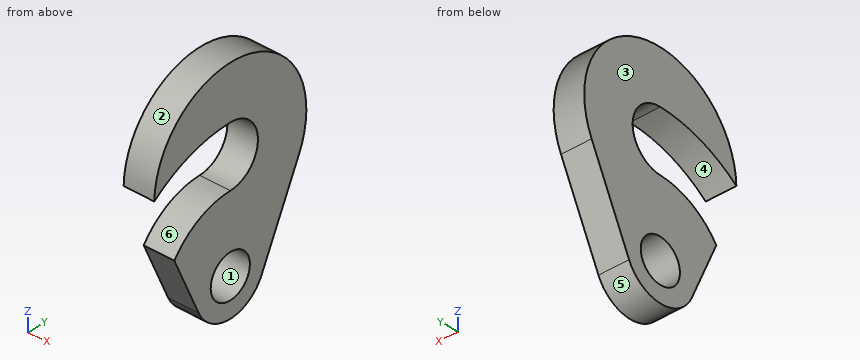
from build123d import *

# Parameters (mm, degrees)
SKETCH1_R           = 8.5
BOSS_EXTRUDE1_DEPTH = 12


with BuildPart() as part:
    # Sketch1 → Boss-Extrude1 (new body)
    with BuildSketch(Plane(origin=(0, 0, 0), x_dir=(0, 0, -1), z_dir=(1, 0, 0))):
        with BuildLine():
            Line((-17.601019721, -24.29411667), (6.119406169, -13.694994273))
            ThreePointArc((6.119406169, -13.694994273), (14.999034519, -0.170186666), (6.428571429, 13.552618544))
            Line((6.428571429, 13.552618544), (-27.857142857, 29.815760796))
            ThreePointArc((-27.857142857, 29.815760796), (-74.109646673, 7.613842033), (-42.75, -32.991476172))
            ThreePointArc((-42.75, -32.991476172), (-51.110175112, -17.428425058), (-54, 0))
            ThreePointArc((-54, 0), (-42, 12), (-30, 0))
            ThreePointArc((-30, 0), (-26.721064646, -13.637620914), (-17.601019721, -24.29411667))
        make_face()
        Circle(SKETCH1_R, mode=Mode.SUBTRACT)
    extrude(amount=BOSS_EXTRUDE1_DEPTH)


solid = part.part
Build history of the part. All positions in model axes, mm. Face numbers are marked on the shaded views. A direction names the side the tool comes from. Round coordinates to 2 decimals unless told otherwise and drop trailing zeros. Write each loop counter-clockwise with the first axis right and the second up, starting at its lowest first coordinate (ties: lowest second). Pieces come first, ordered by that corner, then holes. Notation, with made-up numbers: (-31.75, 69.25) -> (-4.75, 69.25) arc R15 ccw to (-4.75, 77.25) -> close; hole circle Ø8 at (83.5, 67.5). An arc over 180 degrees is marked (long way). Write item = value, one per line.
(1) Two-plate mould, pull along Y, no slides. Class the marked faces 1, 2 and 3: pulls with the +Y half, pulls with the -Y half, needs draft (parallel to the pull), parting line crosses it, or undercut.
Answer:
face_1 = undercut
face_2 = parting line crosses it
face_3 = needs draft
(2) Band-saw the part on B-B (z = 0). Give the cut face in (x, y).
Answer:
outline = (0, -16.43) -> (12, -16.43) -> (12, -8.5) -> (0, -8.5) -> close; (0, 8.5) -> (12, 8.5) -> (12, 16.6) -> (0, 16.6) -> close
(3) Band-saw the part on C-C (y = -9.5). Give the cut face in (x, z), then the cut area to 3 significant figures.
Answer:
outline = (0, -11.61) -> (12, -11.61) -> (12, 28.46) -> (0, 28.46) -> close; (0, 53.16) -> (12, 53.16) -> (12, 73.6) -> (0, 73.6) -> close
area = 726 mm2
(4) Band-saw the part on D-D (y = 21). Give the cut face in (x, z), then the cut area to 3 significant figures.
Answer:
outline = (0, 9.27) -> (12, 9.27) -> (12, 67.46) -> (0, 67.46) -> close
area = 698 mm2
(5) Probe L1, parallel to Y at x = 9.5, z = 0; L2, parallel to Z at x = 1, y = 9.5; L3, parallel to Z at x = 6.25, y = -18. List the from-to ranges inside material, lowest first.
Answer:
L1 = -16.43 to -8.5, 8.5 to 16.6
L2 = -11.61 to 34.67, 49.33 to 73.6
L3 = 3.52 to 24, 50.91 to 69.66
(6) Flat gauge pins, fed straight in: pin 1 (3 mm diameter, centred on x = 9, z = 63.5, fed in from +Y); pin 2 (5 mm diameter, centred on x = 10, y = 6.5, fed in from -Z); pin 3 (5 mm diameter, centred on x = 3.5, y = 20.5, fed in from +Z); pin 4 (10 mm diameter, centred on y = 0, z = 0, fed in from +X). Where does each tip first touch, or does it go through?
Answer:
pin_1 = 26.25
pin_2 = -14.46
pin_3 = 69.66
pin_4 = through
(7) Band-saw the part on A-A (x = 9.5). Give the cut face in (y, z) (3 decimals).
Answer:
outline = (-32.991, 42.75) arc R54 cw to (0, 54) arc R12 cw to (0, 30) arc R30 ccw to (-24.294, 17.601) -> (-13.695, -6.119) arc R15 ccw to (13.553, -6.429) -> (29.816, 27.857) arc R33 ccw (long way) to start; hole circle Ø17 at (0, 0)
(8) Tool access for the marked faces 4, 5 and 6: list every direction of +Z, -Z, +X, -X, +Y, -Y with a clear straight run to the whole face (end or side of a thin tool).
Answer:
face_4 = +X, -X
face_5 = -Z, +X, -X
face_6 = +X, -X, -Y
